Geometry check sheet. Reference: drawing and pictorial views, mm from the part's lowest x, y, z. Coordinates: 2 decimals unless noted, no trailing zeros. Write each loop counter-clockwise with the first axis right and the second up, starting at its lowest first coordinate (ties: lowest second). Pieces come first, ordered by that corner, then holes. Notation, with made-up numbers: (-4, 76.5) -> (47, 76.5) arc R4 ccw to (47, 82.5) -> close; hole circle Ø7 at (4.25, 49.25). An arc over 180 degrees is marked (long way). Use a Markdown table: item, result.
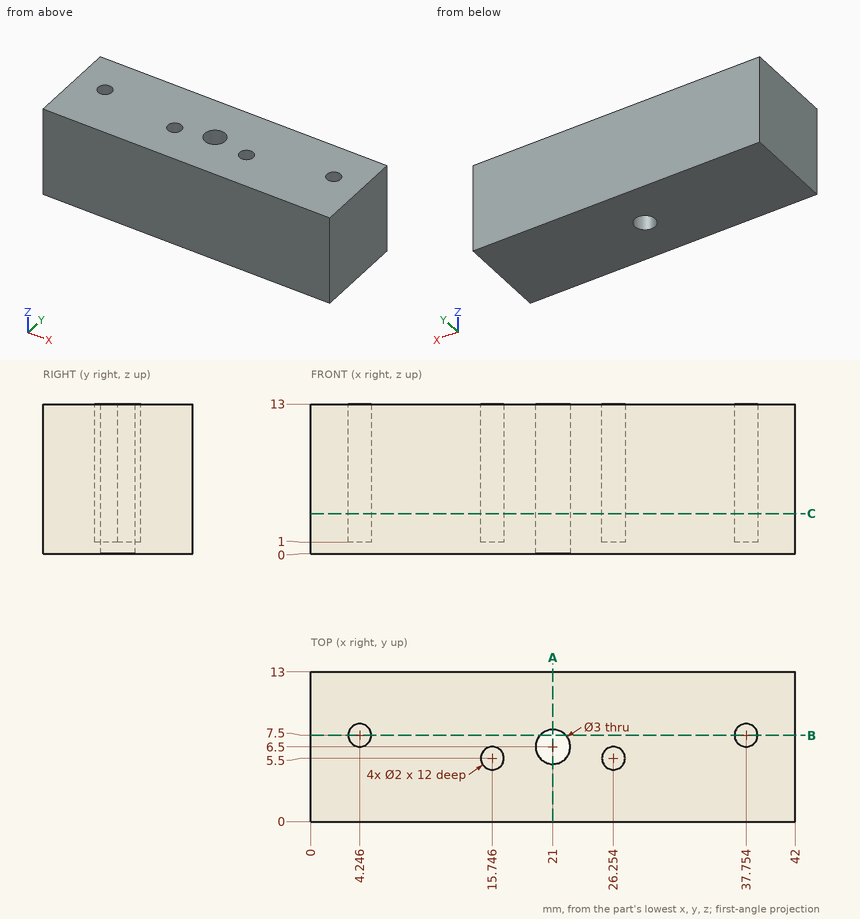
Item 1: Section check C-C on z = 3.5. Record the boundary of the cut face in (x, y).
Answer block:
| item | result |
|---|---|
| outline | (0, 0) -> (42, 0) -> (42, 13) -> (0, 13) -> close; hole circle Ø2 at (4.25, 7.5); hole circle Ø2 at (15.75, 5.5); hole circle Ø3 at (21, 6.5); hole circle Ø2 at (26.25, 5.5); hole circle Ø2 at (37.75, 7.5) |
Item 2: Section check B-B on y = 7.5. Record the boundary of the cut face in (x, z), then the cut area to 3 significant figures.
Answer block:
| item | result |
|---|---|
| outline | (0, 0) -> (19.88, 0) -> (19.88, 13) -> (5.25, 13) -> (5.25, 1) -> (3.25, 1) -> (3.25, 13) -> (0, 13) -> close; (22.12, 0) -> (42, 0) -> (42, 13) -> (38.75, 13) -> (38.75, 1) -> (36.75, 1) -> (36.75, 13) -> (22.12, 13) -> close |
| area | 469 mm^2 |
Item 3: Thickness scan on L1, parallel to Y at x = 25.5, z = 11.75; L2, parallel to Y at x = 3.5, z = 7.75 (1 decimal). Record the ranges inside material, lowest first. Write a range as [from, to].
Answer block:
| item | result |
|---|---|
| L1 | y = [0, 4.84], [6.16, 13] |
| L2 | y = [0, 6.8], [8.2, 13] |
Item 4: Section check A-A on x = 21. Record the boundary of the cut face in (y, z).
Answer block:
| item | result |
|---|---|
| outline | (0, 0) -> (5, 0) -> (5, 13) -> (0, 13) -> close; (8, 0) -> (13, 0) -> (13, 13) -> (8, 13) -> close |
Item 5: Depth check by flat-ended pin: P1, Ø0.6, axis at x = 16, y = 6, coming from the +Z side; P2, Ø2.5, axis at x = 21, y = 6.5, coming from the +Z side. Enter the tip coordinate at first touch or a pass-through.
Answer block:
| item | result |
|---|---|
| P1 | stops at z = 1 |
| P2 | passes through |
